```python
from build123d import *

# Parameters (mm, degrees)
EXTRUDE_1_DEPTH          = 600
CUT_EXTRUDE_1_DEPTH      = 300
CUT_EXTRUDE_2_DEPTH      = 310
CUT_EXTRUDE_2_DEPTH_BACK = 150
CUT_EXTRUDE_3_DEPTH      = 100
EXTRUDE_2_DEPTH          = 20


with BuildPart() as part:
    # Эскиз1 → Бобышка-Вытянуть1 (new body)
    with BuildSketch(Plane(origin=(0, 0, 0), x_dir=(1, 0, 0), z_dir=(0, 1, 0))):
        Polygon((-900, 950), (900, 950), (850, 0), (-850, 0), align=None)
    extrude(amount=EXTRUDE_1_DEPTH)

    # Эскиз3 → Вырез-Вытянуть1 (cut)
    with BuildSketch(Plane(origin=(0, 600, 0), x_dir=(1, 0, 0), z_dir=(0, 1, 0))):
        Polygon((-830.084404496, 896.603685423), (830.084404496, 896.603685423), (785, 40), (-785, 40), align=None)
    extrude(amount=-CUT_EXTRUDE_1_DEPTH, mode=Mode.SUBTRACT)

    # Эскиз4 → Вырез-Вытянуть2 (cut, two sides)
    with BuildSketch(Plane(origin=(0, 300, 0), x_dir=(1, 0, 0), z_dir=(0, 1, 0))) as cut_extrude_2_sk:
        Polygon((-830.084404496, 896.603685423), (830.084404496, 896.603685423), (815.955318169, 628.151045218), (709.135748769, 628.151045218), (695.096165279, 361.398958916), (801.91573468, 361.398958916), (785, 40), (700, 40), (700, 0), (-700, 0), (-700, 40), (-785, 40), (-801.91573468, 361.398958916), (-685.814283751, 361.398958916), (-699.85386724, 628.151045218), (-815.955318169, 628.151045218), align=None)
    extrude(amount=CUT_EXTRUDE_2_DEPTH, mode=Mode.SUBTRACT)
    extrude(cut_extrude_2_sk.sketch, amount=-CUT_EXTRUDE_2_DEPTH_BACK, mode=Mode.SUBTRACT)

    # Эскиз5 → Вырез-Вытянуть3 (cut)
    with BuildSketch(Plane(origin=(0, 150, 0), x_dir=(1, 0, 0), z_dir=(0, 1, 0))):
        Polygon((-830.084404496, 896.603685423), (-815.955318169, 628.151045218), (-701.325281658, 628.151045218), (-687.285698169, 361.398958916), (-801.91573468, 361.398958916), (-785, 40), (785, 40), (801.91573468, 361.398958916), (694.58093137, 361.398958916), (708.814837931, 628.151045218), (815.955318169, 628.151045218), (830.084404496, 896.603685423), align=None)
    extrude(amount=-CUT_EXTRUDE_3_DEPTH, mode=Mode.SUBTRACT)

    # Эскиз6 → Бобышка-Вытянуть2 (add)
    with BuildSketch(Plane(origin=(0, 600, 0), x_dir=(1, 0, 0), z_dir=(0, 1, 0))):
        Polygon((-900, 950), (-850, 0), (-700, 0), (-721.056000817, 400.064015528), (721.056000817, 400.064015528), (700, 0), (849.722904554, -5.264813473), (900, 950), align=None)
    extrude(amount=EXTRUDE_2_DEPTH)


solid = part.part
```
Here's how the part is built. I have some questions about the finished solid (model axes, mm). A direction names the side the tool comes from. Give positions to 0.01 mm unless a question says otherwise; leave off trailing zeros. Loops run counter-clockwise (first coordinate to the right, second up) from the corner with the lowest first, then second, coordinate; pieces in that order, holes last. Notation, with made-up numbers: M 81,25 L 110,25 A10 cw 110,31 Z; hole C 6,25.25 d3. An arc over 180 degrees is marked long. Return JSON: item names as keys, results as strings.
Item 1: Thinking about a two-plate mould opening in Z: for faces 4 (the flat face through (700, 372, -20)), 5 (the flat face through (-12, 99, 0)), 6 (the flat face through (-692.736, 226.05, -492.908)), 7 (the flat face through (-694.4, 100.7, -496.6)), which applies, released by +Z, released by -Z, zero draft, split by the parting line, or undercut?
A:
{"face 4": "zero draft", "face 5": "released by +Z", "face 6": "undercut", "face 7": "undercut"}
Item 2: Imagine slicing it at C-C on z = -768.5. List the corners of the cut face in (x, y) for me.
A:
{"outline": "M -890.45,0 L 890.45,0 L 890.45,620 L -890.45,620 Z; hole M -823.34,50 L 823.34,50 L 823.34,600 L -823.34,600 Z"}
Item 3: Imagine slicing it at A-A on y = 101.5. List the corners of the cut face in (x, z) for me.
A:
{"outline": "M -900,-950 L 900,-950 L 850,0 L -850,0 Z; hole M -830.08,-896.6 L 830.08,-896.6 L 815.96,-628.15 L 708.81,-628.15 L 694.58,-361.4 L 801.92,-361.4 L 785,-40 L -785,-40 L -801.92,-361.4 L -687.29,-361.4 L -701.33,-628.15 L -815.96,-628.15 Z"}
Item 4: I'm going to push flat-ended pins straight in: pin 1 Ø1 at (y, z) = (227, -721) entering from -X; pin 2 Ø1.5 at (x, y) = (627.5, 125) entering from +Z; pin 3 Ø20 at (x, z) = (-91.5, -25.5) entering from +Y. Where does each tip first touch, or does it pass through?
A:
{"pin 1": "stops at x = -887.97", "pin 2": "stops at z = 0", "pin 3": "stops at y = 150"}
Item 5: Imagine slicing it at B-B on y = 263. List the corners of the cut face in (x, z) for me.
A:
{"outline": "M -900,-950 L 900,-950 L 850,0 L 700,0 L 700,-40 L 785,-40 L 801.92,-361.4 L 695.1,-361.4 L 709.14,-628.15 L 815.96,-628.15 L 830.08,-896.6 L -830.08,-896.6 L -815.96,-628.15 L -699.85,-628.15 L -685.81,-361.4 L -801.92,-361.4 L -785,-40 L -700,-40 L -700,0 L -850,0 Z"}
Item 6: Please list where these lines run through material, in increasing order: line 1 (Z direction, x = 741.5, y = 113.5); line 2 (Y direction, x = 437, z = -813); line 3 (Z direction, x = 154, y = 85).
A:
{"line 1": "z = -950 to -896.6, -628.15 to -361.4, -40 to 0", "line 2": "y = 0 to 50, 600 to 620", "line 3": "z = -950 to -896.6, -40 to 0"}
Item 7: On a 3-axis mill with a long thin cutter (end or side, diameter ignored), from which of +Z, -Z, +X, -X, +Y, -Y can I reach the whole of each face in a straight line? I mean faces 1 (the flat face through (763, 177, -628.151)), 2 (the flat face through (-700, 372, -20)), 3 (the flat face through (874.51, 305.66, -465.68)). Say none if no direction works.
A:
{"face 1": "none", "face 2": "+Z, +Y", "face 3": "+Z, +X, +Y, -Y"}
Item 8: Imagine slicing it at D-D on x = -29. List the corners of the cut face in (y, z) for me, then the cut area to 3 significant figures.
A:
{"outline": "M 0,-950 L 620,-950 L 620,-400.06 L 600,-400.06 L 600,-896.6 L 50,-896.6 L 50,-40 L 150,-40 L 150,0 L 0,0 Z", "area": "91,900 mm^2"}
